```python
from build123d import *

# Parameters (mm, degrees)
F1_DEPTH = 28
F2_R     = 1.1
F3_DEPTH = 32.301
F4_R     = 1.1
F5_DEPTH = 1.5
F6_W     = 1.5
F6_H     = 86.945
F7_DEPTH = 32.3
F8_R     = 1.1
F9_DEPTH = 32.301


with BuildPart() as f1:
    # F0 (on Front) → F1 (new body)
    with BuildSketch(Plane.XZ):
        Polygon((0, 86.945), (0, 0), (1.5, 0), (1.5, 85.445), (30.8, 85.445), (30.8, 0), (32.3, 0), (32.3, 86.945), align=None)
    extrude(amount=F1_DEPTH)

    # F2 (on face) → F3 (cut, through all)
    with BuildSketch(Plane(origin=(0, 0, 0), x_dir=(0, -1, 0), z_dir=(-1, 0, 0))):
        with BuildLine():
            Line((18, 0), (18, 2))
            ThreePointArc((18, 2), (14, 6), (10, 2))
            Line((10, 2), (10, 0))
            Line((10, 0), (18, 0))
        make_face()
        with Locations((20.22254, 2)):
            Circle(F2_R)
        with Locations((18.4, 6.4)):
            Circle(F2_R)
        with Locations((14, 8.22254)):
            Circle(F2_R)
        with Locations((9.6, 6.4)):
            Circle(F2_R)
        with Locations((7.77746, 2)):
            Circle(F2_R)
    extrude(amount=-F3_DEPTH, mode=Mode.SUBTRACT)

    # F4 (on face) → F5 (cut, through all)
    with BuildSketch(Plane.XY.offset(86.945)):
        with Locations((6.15, -4)):
            Circle(F4_R)
        with Locations((26.15, -4)):
            Circle(F4_R)
        with Locations((6.15, -24)):
            Circle(F4_R)
        with Locations((26.15, -24)):
            Circle(F4_R)
    extrude(amount=-F5_DEPTH, mode=Mode.SUBTRACT)

    # F6 (on face) → F7 (join)
    with BuildSketch(Plane.YZ.offset(32.3)):
        with Locations((-28.75, 43.4725)):
            Rectangle(F6_W, F6_H)
    extrude(amount=-F7_DEPTH)

    # F8 (on face) → F9 (cut, through all)
    with BuildSketch(Plane.YZ.offset(32.3)):
        Polygon((0, 86.945), (-29.5, 86.945), (-29.5, 85.445), (-18, 85.445), (-10, 85.445), (0, 85.445), align=None)
        with BuildLine():
            Line((-10, 85.445), (-18, 85.445))
            Line((-18, 85.445), (-18, 83.445))
            ThreePointArc((-18, 83.445), (-14, 79.445), (-10, 83.445))
            Line((-10, 83.445), (-10, 85.445))
        make_face()
        with Locations((-18.4, 6.4)):
            Circle(F8_R)
        with Locations((-14, 8.22254)):
            Circle(F8_R)
        with Locations((-9.6, 6.4)):
            Circle(F8_R)
        with Locations((-7.77746, 2)):
            Circle(F8_R)
        with Locations((-20.22254, 2)):
            Circle(F8_R)
        with Locations((-9.6, 79.045)):
            Circle(F8_R)
        with Locations((-18.4, 79.045)):
            Circle(F8_R)
        with Locations((-7.77746, 83.445)):
            Circle(F8_R)
        with Locations((-14, 77.22246)):
            Circle(F8_R)
        with Locations((-20.22254, 83.445)):
            Circle(F8_R)
    extrude(amount=-F9_DEPTH, mode=Mode.SUBTRACT)


solid = f1.part
```
Model file for the job. Use its own axes, mm. A direction names the side the tool comes from. Round coordinates to 2 decimals unless told otherwise and drop trailing zeros. Write each loop counter-clockwise with the first axis right and the second up, starting at its lowest first coordinate (ties: lowest second). Pieces come first, ordered by that corner, then holes. Notation, with made-up numbers: (-28.5, 36) -> (-22.5, 36) arc R28 ccw to (-22.5, 62) -> close; hole circle Ø4 at (64, 41). An arc over 180 degrees is marked (long way). Answer as CSV lines item,"result".
1. Slice it at C-C, the plane x = 16. List the corners of the cut face in (y, z) (3 decimals).
Resolved:
outline,"(-29.5, 0) -> (-28, 0) -> (-28, 85.445) -> (-29.5, 85.445) -> close"
2. Drill centre lines: line 1 (Y direction, x = 0.65, z = 6.4); line 2 (Y direction, x = 1, z = 2); line 3 (X direction, y = -26, z = 39). Where is each one in solid material? Low to high.
Resolved:
line 1,"-29.5 to -19.5, -17.3 to -10.7, -8.5 to 0"
line 2,"-29.5 to -21.32, -19.12 to -18, -10 to -8.88, -6.68 to 0"
line 3,"0 to 1.5, 30.8 to 32.3"
3. Pin check, flat tips, straight feed: pin 1 Ø3 at (y, z) = (-14, 8.22) entering from +X; pin 2 Ø6 at (x, z) = (5, 48.5) entering from +Y. Stop position of each tip, or through.
Resolved:
pin 1,"x = 32.3"
pin 2,"y = -28"
4. Mould opens along Z. For faces 1 (the face through (16.2, -28.5, 85.445)), 2 (the face through (0.76, -14.87, 76.55)), 3 (the face through (1, -14, 6)), 4 (the face through (1, -10, 84)) say: +Z half, -Z half, draft (parallel to the pull), parting line (faces both ways), or undercut.
Resolved:
face 1,"+Z half"
face 2,"undercut"
face 3,"-Z half"
face 4,"draft"
5. Slice it at B-B, the plane z = 47. List the corners of the cut face in (x, y).
Resolved:
outline,"(0, -29.5) -> (32.3, -29.5) -> (32.3, 0) -> (30.8, 0) -> (30.8, -28) -> (1.5, -28) -> (1.5, 0) -> (0, 0) -> close"
6. Slice it at A-A, the plane y = -2.5. List the corners of the cut face in (x, z) (3 decimals).
Resolved:
outline,"(0, 0) -> (1.5, 0) -> (1.5, 85.445) -> (0, 85.445) -> close; (30.8, 0) -> (32.3, 0) -> (32.3, 85.445) -> (30.8, 85.445) -> close"
7. Tool access for faces 5 (the face through (1, -18, 84)), 6 (the face through (32, -5, 85.445)), 7 (the face through (1.5, -14, 42)): list every direction of +Z, -Z, +X, -X, +Y, -Y with a clear straight run to the whole face (end or side of a thin tool).
Resolved:
face 5,"+Z, +X, -X"
face 6,"+Z, +X, -X, +Y, -Y"
face 7,"+Z, -Z, +Y"
